Here's how the part is built. I have some questions about the finished solid (model axes, mm). A direction names the side the tool comes from. Round coordinates to 2 decimals unless told otherwise and drop trailing zeros. Order: outer loops, then holes, each group sorted by start corner. A loop starts at its lowest first (then second) coordinate and runs counter-clockwise, first axis right, second up.
Autodesk Inventor part; units mm, degrees
ref_plane "YZ Plane" through (0, 0, 0) normal (1, 0, 0) x (0, 1, 0)
ref_plane "XZ Plane" through (0, 0, 0) normal (0, 1, 0) x (-1, 0, 0)
ref_plane "XY Plane" through (0, 0, 0) normal (0, 0, 1) x (1, 0, 0)
sketch "Sketch1" plane through (0, 0, 0) normal (0, 0, 1) x (1, 0, 0)
  line L0 (-12.5, 9.5) -> (-12.5, -14.5) construction
  line L1 (-15.5, -14.5) -> (-15.5, 9.5) construction
  line L2 (-12.5, -2.5) -> (-15.5, -2.5) construction
  line L3 (26, -17.5) -> (-54, -17.5)
  line L4 (-54, -17.5) -> (-54, 12.5)
  line L5 (-54, 12.5) -> (26, 12.5)
  line L6 (26, 12.5) -> (26, -17.5)
  line L7 (26, -17.5) -> (-54, 12.5) construction
  line L8 (-54, -17.5) -> (26, 12.5) construction
  line L9 (-12.5, -14.5) -> (12.5, -14.5) construction
  line L10 (12.5, -14.5) -> (12.5, 9.5) construction
  line L11 (12.5, 9.5) -> (-12.5, 9.5) construction
  line L12 (-15.5, 9.5) -> (-40.5, 9.5) construction
  line L13 (-40.5, 9.5) -> (-40.5, -14.5) construction
  line L14 (-40.5, -14.5) -> (-15.5, -14.5) construction
  line L15 (-8.7, -9.1) -> (-8.7, -9.9) construction
  line L16 (-8.7, -9.9) -> (-7.48, -9.9) construction
  line L17 (-7.48, -9.9) -> (-7.48, -9.1) construction
  line L18 (-7.48, -9.1) -> (-8.7, -9.1) construction
  circle A0 centre (-10.5, -12.5) radius 1.05
  circle A1 centre (-10.5, 0) radius 1.05
  circle A2 centre (10.5, 0) radius 1.05
  circle A3 centre (10.5, -12.5) radius 1.05
  circle A4 centre (-17.5, -12.5) radius 1.05
  circle A5 centre (-17.5, 0) radius 1.05
  circle A6 centre (-38.5, -12.5) radius 1.05
  circle A7 centre (-38.5, 0) radius 1.05
  line L19 (5.5, -14.5) -> (-5.5, -14.5)
  line L20 (5.5, 6.5) -> (5.5, -14.5)
  line L21 (-5.5, -10.5) -> (-9.45, -10.5)
  line L22 (-5.5, -8.5) -> (-9.45, -8.5)
  line L23 (-9.45, -10.5) -> (-9.45, -8.5)
  line L24 (-5.5, -14.5) -> (-5.5, -10.5)
  line L25 (-5.5, -8.5) -> (-5.5, 6.5)
  line L26 (-35.3, -11.5) -> (-35.3, 8.5)
  line L27 (-20.7, 8.5) -> (-20.7, -11.5)
  line L28 (5.5, 6.5) -> (-5.5, 6.5)
  line L29 (-20.7, -11.5) -> (-35.3, -11.5)
  line L30 (-20.7, 8.5) -> (-35.3, 8.5)
  line L31 (20.75, 12.5) -> (17.75, 12.5)
  line L32 (17.75, 12.5) -> (17.75, -2.5)
  line L33 (17.75, -2.5) -> (20.75, -2.5)
  line L34 (20.75, -2.5) -> (20.75, 12.5)
  line L35 (-14, -17.5) -> (-14, 12.5) construction
  line L36 (-48.75, 12.5) -> (-45.75, 12.5)
  line L37 (-45.75, 12.5) -> (-45.75, -2.5)
  line L38 (-45.75, -2.5) -> (-48.75, -2.5)
  line L39 (-48.75, -2.5) -> (-48.75, 12.5)
  point P0 (0, 0)
  point P1 (-14, -2.5)
  dimension "d0" = 80
  dimension "d1" = 30
  dimension "d2" = 7
  dimension "d4" = 4
  dimension "d6" = 18
  dimension "d7" = 7
  dimension "d8" = 7
  dimension "d9" = 3.05
  dimension "d10" = 3
  dimension "d11" = 5.2
  dimension "d12" = 5.2
  dimension "d13" = 3
  dimension "d14" = 3
  dimension "d15" = 1
  dimension "d16" = 15
  dimension "d17" = 5.25
  dimension "d18" = 13.5
  dimension "d19" = 3
extrude "Extrusion1" add sketch "Sketch1" along normal blind 3 contours L3 L4 L5 L39 L38 L37 L32 L33 L34 L6
properties part number "Camera bracket"
1) If we section it at C-C (y = -12.5): Write out the boundary of the cut face in (x, z).
2) I need wall thicknesses on line 1 (X direction, y = 10.25, z = 1.5); line 2 (X direction, y = 8, z = 0.25); line 3 (Y direction, x = 10.5, z = 1.8). Which ranges of each line are inside material? Lowest first, please.
3) We'd pull the mould along Y, two halves only. Please class faces 4 (the flat face through (19, -2.5, 1)), 5 (the flat face through (-15, -2, 3)), 6 (the cylindrical face through (-39.55, -12.55, 1.48)), 7 (the flat face through (0, 6.5, 1)): +Y half, -Y half, draft (parallel to the pull), parting line (faces both ways), or undercut.
4) If we section it at A-A (y = -9.5): Write out the boundary of the cut face in (x, z).
5) I'm going to push a flat-ended pin straight in: pin 1 (3.5 mm diameter, centred on x = -10.5, y = -12.5, fed in from -Z). Where does the tip first touch, or does it pass through?
6) If we section it at B-B (x = -6.5): Write out the boundary of the cut face in (y, z), plus the area to 3 significant figures.
7) If we section it at D-D (x = 10.5): Write out the boundary of the cut face in (y, z).
8) For faces 1 (the flat face through (-48.75, 5, 1)), 2 (the flat face through (-15, -2, 0)), 3 (the flat face through (-28, -11.5, 1)), which set-ups out of +Z, -Z, +X, -X, +Y, -Y let a thin tool reach every point of the face, with its end or its side?
Solutions:
1. outline: (-54, 0) - (-39.55, 0) - (-39.55, 3) - (-54, 3) - close; (-37.45, 0) - (-18.55, 0) - (-18.55, 3) - (-37.45, 3) - close; (-16.45, 0) - (-11.55, 0) - (-11.55, 3) - (-16.45, 3) - close; (-9.45, 0) - (-5.5, 0) - (-5.5, 3) - (-9.45, 3) - close; (5.5, 0) - (9.45, 0) - (9.45, 3) - (5.5, 3) - close; (11.55, 0) - (26, 0) - (26, 3) - (11.55, 3) - close
2. line 1: x = -54 to -48.75, -45.75 to 17.75, 20.75 to 26
2. line 2: x = -54 to -48.75, -45.75 to -35.3, -20.7 to 17.75, 20.75 to 26
2. line 3: y = -17.5 to -13.55, -11.45 to -1.05, 1.05 to 12.5
3. face 4: +Y half
3. face 5: draft
3. face 6: undercut
3. face 7: undercut
4. outline: (-54, 0) - (-35.3, 0) - (-35.3, 3) - (-54, 3) - close; (-20.7, 0) - (-9.45, 0) - (-9.45, 3) - (-20.7, 3) - close; (5.5, 0) - (26, 0) - (26, 3) - (5.5, 3) - close
5. pin 1: stops at z = 0
6. outline: (-17.5, 0) - (-10.5, 0) - (-10.5, 3) - (-17.5, 3) - close; (-8.5, 0) - (12.5, 0) - (12.5, 3) - (-8.5, 3) - close
6. area: 84.0 mm2
7. outline: (-17.5, 0) - (-13.55, 0) - (-13.55, 3) - (-17.5, 3) - close; (-11.45, 0) - (-1.05, 0) - (-1.05, 3) - (-11.45, 3) - close; (1.05, 0) - (12.5, 0) - (12.5, 3) - (1.05, 3) - close
8. face 1: +Z, -Z, +Y
8. face 2: -Z, +X, -X, +Y, -Y
8. face 3: +Z, -Z
